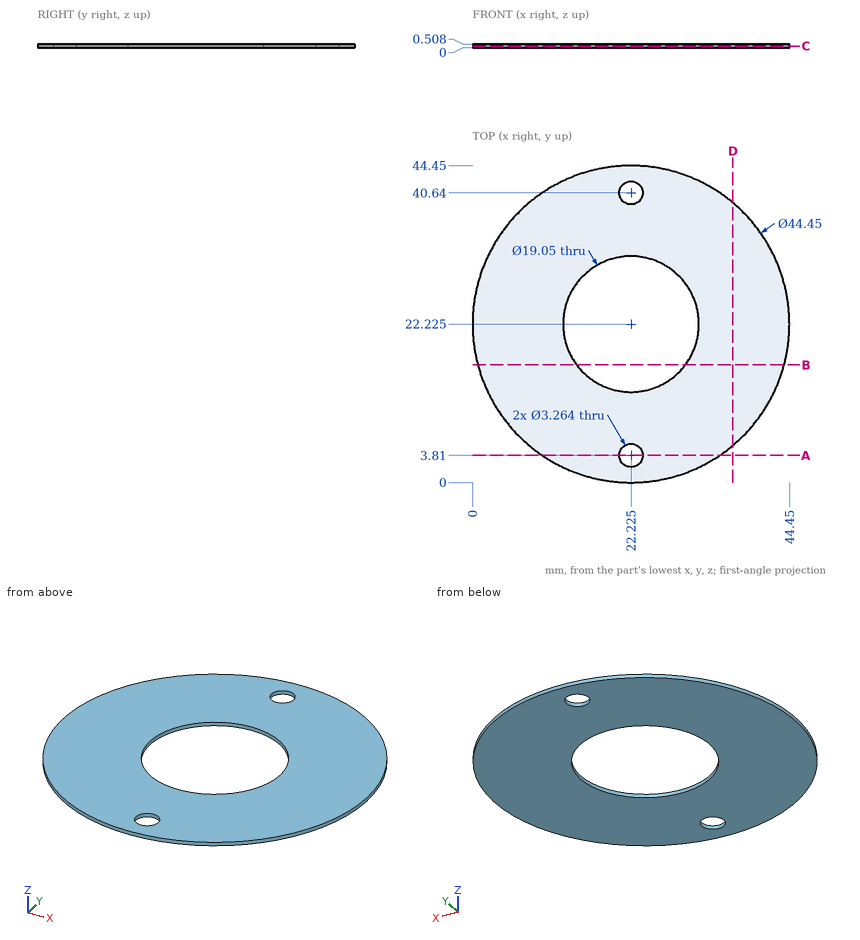
Print and shaded views of the part. All mm, measured from the part's lowest x, y and z. Give positions to 0.01 mm unless a question says otherwise; leave off trailing zeros. Order: outer loops, then holes, each group sorted by start corner. A loop starts at its lowest first (then second) coordinate and runs counter-clockwise, first axis right, second up. Notation, with made-up numbers: M 51.25,21 L 74.25,21 A29 ccw 74.25,48 Z; hole C 5.5,33 d11. An arc over 180 degrees is marked long. Use one line per item in the form item = value.
Q1. Slice it at A-A, the plane y = 3.81. Write the cut outline in (x, z), and give its area (3 significant figures).
Conclusion:
outline = M 9.78,0 L 20.59,0 L 20.59,0.51 L 9.78,0.51 Z; M 23.86,0 L 34.67,0 L 34.67,0.51 L 23.86,0.51 Z
area = 11.0 mm2
Q2. Slice it at B-B, the plane y = 16.5. Write the cut outline in (x, z), and give its area (3 significant figures).
Conclusion:
outline = M 0.75,0 L 14.61,0 L 14.61,0.51 L 0.75,0.51 Z; M 29.84,0 L 43.7,0 L 43.7,0.51 L 29.84,0.51 Z
area = 14.1 mm2
Q3. Pin check, flat tip, straight feed: P1, Ø2, axis at x = 22.225, y = 40.64, coming from the -Z side. Stop position of the tip, or through.
Conclusion:
P1 = through
Q4. Wall check: probe 1 along X at (y, z) = (22, 0.1); probe 2 along Y at (x, z) = (22, 0.15); probe 3 along X at (y, z) = (17, 0.1). Give the ranges that are in metal, low to high.
Conclusion:
probe_1 = 0 to 12.7, 31.75 to 44.45
probe_2 = 0 to 2.19, 5.43 to 12.7, 31.75 to 39.02, 42.26 to 44.45
probe_3 = 0.62 to 14.26, 30.19 to 43.83
Q5. Slice it at C-C, the plane z = 0.2. Write the cut outline in (x, y) (3 decimals), and give its area (3 significant figures).
Conclusion:
outline = C 22.225,22.225 d44.45; hole C 22.225,22.225 d19.05; hole C 22.225,3.81 d3.264; hole C 22.225,40.64 d3.264
area = 1,250 mm2
Q6. Slice it at D-D, the plane x = 36.5. Write the cut outline in (y, z), and give its area (3 significant figures).
Conclusion:
outline = M 5.19,0 L 39.26,0 L 39.26,0.51 L 5.19,0.51 Z
area = 17.3 mm2
